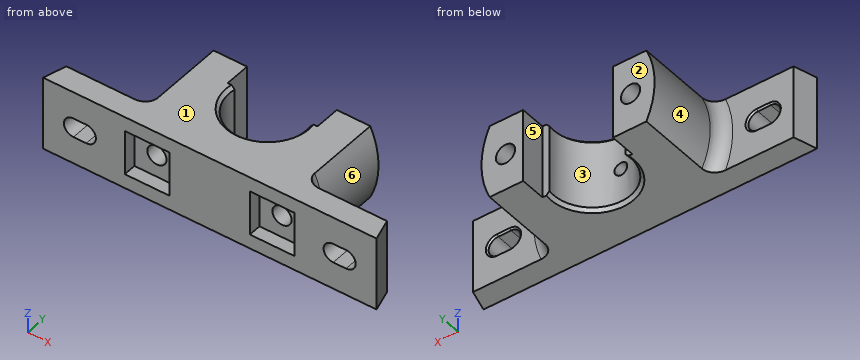
```python
from build123d import *

# Parameters (mm, degrees)
BOSS_EXTRUDE1_DEPTH = 23
BOSS_EXTRUDE2_DEPTH = 54
CUT_EXTRUDE1_DEPTH  = 47
SKETCH4_R           = 6
CUT_EXTRUDE2_DEPTH  = 69
SKETCH5_W           = 28
SKETCH5_H           = 28
CUT_EXTRUDE3_DEPTH  = 8
CUT_EXTRUDE4_DEPTH  = 15
SKETCH7_R           = 4
CUT_EXTRUDE5_DEPTH  = 54
FILLET1_R           = 8
CHAMFER1_SIZE       = 2
CHAMFER2_SIZE       = 1


with BuildPart() as part:
    # Sketch1 → Boss-Extrude1 (new body, symmetric)
    with BuildSketch(Plane.XY):
        Polygon((-104, 0), (104, 0), (99.985564599, 14), (-99.985564599, 14), align=None)
    extrude(amount=BOSS_EXTRUDE1_DEPTH, both=True)

    # Sketch2 → Boss-Extrude2 (add)
    with BuildSketch(Plane(origin=(0, 14, 0), x_dir=(1, 0, 0), z_dir=(0, 1, 0))):
        with BuildLine():
            Line((48.856934001, 23), (-48.856934001, 23))
            ThreePointArc((-48.856934001, 23), (-54, 0), (-48.856934001, -23))
            Line((-48.856934001, -23), (48.856934001, -23))
            ThreePointArc((48.856934001, -23), (54, 0), (48.856934001, 23))
        make_face()
    extrude(amount=BOSS_EXTRUDE2_DEPTH)

    # Sketch3 → Cut-Extrude1 (cut, through all)
    with BuildSketch(Plane.XY.offset(23)):
        with BuildLine():
            Line((-28, 68), (-28, 52))
            Line((-28, 52), (-23.664319132, 52))
            ThreePointArc((-23.664319132, 52), (0, 24), (23.664319132, 52))
            Line((23.664319132, 52), (28, 52))
            Line((28, 52), (28, 68))
            Line((28, 68), (-28, 68))
        make_face()
    extrude(amount=-CUT_EXTRUDE1_DEPTH, mode=Mode.SUBTRACT)

    # Sketch4 → Cut-Extrude2 (cut, through all)
    with BuildSketch(Plane(origin=(0, 68, 0), x_dir=(1, 0, 0), z_dir=(0, 1, 0))):
        with Locations(Location((-39, 0, 0), (0, 0, 270))):  # turned: the seam where the file's is
            Circle(SKETCH4_R)
        with Locations(Location((39, 0, 0), (0, 0, 270))):  # turned: the seam where the file's is
            Circle(SKETCH4_R)
    extrude(amount=-CUT_EXTRUDE2_DEPTH, mode=Mode.SUBTRACT)

    # Sketch5 → Cut-Extrude3 (cut)
    with BuildSketch(Plane.XZ):
        with Locations((-39, 0)):
            Rectangle(SKETCH5_W, SKETCH5_H)
        with Locations((39, 0)):
            Rectangle(SKETCH5_W, SKETCH5_H)
    extrude(amount=-CUT_EXTRUDE3_DEPTH, mode=Mode.SUBTRACT)

    # Sketch6 → Cut-Extrude4 (cut, through all)
    with BuildSketch(Plane(origin=(0, 14, 0), x_dir=(1, 0, 0), z_dir=(0, 1, 0))):
        with BuildLine():
            Line((-85, 6), (-77, 6))
            ThreePointArc((-77, 6), (-71, 0), (-77, -6))
            Line((-77, -6), (-85, -6))
            ThreePointArc((-85, -6), (-91, 0), (-85, 6))
        make_face()
    cut_extrude4 = extrude(amount=-CUT_EXTRUDE4_DEPTH, mode=Mode.SUBTRACT)

    # Mirror1: Cut-Extrude4 across plane
    add(cut_extrude4.mirror(Plane(origin=(0, 0, 0), x_dir=(0, 0, 1), z_dir=(1, 0, 0))), mode=Mode.SUBTRACT)

    # Sketch7 → Cut-Extrude5 (cut)
    with BuildSketch(Plane(origin=(0, 68, 0), x_dir=(1, 0, 0), z_dir=(0, 1, 0))):
        with Locations(Location((0, 0, 0), (0, 0, 270))):  # turned: the seam where the file's is
            Circle(SKETCH7_R)
    extrude(amount=-CUT_EXTRUDE5_DEPTH, mode=Mode.SUBTRACT)

    # Fillet1
    fillet1_edges = [part.edges().sort_by_distance(p)[0] for p in [
        (54, 14, 0),
        (-54, 14, 0),
    ]]
    fillet(fillet1_edges, radius=FILLET1_R)

    # Chamfer1
    chamfer1_edges = [part.edges().sort_by_distance(p)[0] for p in [
        (0, 24, -23),
        (0, 24, 23),
    ]]
    chamfer(chamfer1_edges, length=CHAMFER1_SIZE)

    # Chamfer2
    chamfer2_edges = [part.edges().sort_by_distance(p)[0] for p in [
        (91, 14, 0),
        (81, 14, 6),
        (71, 14, 0),
        (81, 14, -6),
        (-91, 14, 0),
        (-81, 14, 6),
        (-71, 14, 0),
        (-81, 14, -6),
    ]]
    chamfer(chamfer2_edges, length=CHAMFER2_SIZE)


solid = part.part
```
The listing builds one solid part. Answer for the finished solid, in the listing's coordinates (mm). Face numbers are marked on the shaded views. A direction names the side the tool comes from. Round coordinates to 2 decimals unless told otherwise and drop trailing zeros. Write each loop counter-clockwise with the first axis right and the second up, starting at its lowest first coordinate (ties: lowest second). Pieces come first, ordered by that corner, then holes. Notation, with made-up numbers: (-16.5, -22) -> (15.5, -22) arc R26 cw to (15.5, 2) -> close; hole circle Ø5 at (-34.75, -3.75). An arc over 180 degrees is marked (long way). Write item = value, one per line.
1) Which of the six approach directions +Z, -Z, +X, -X, +Y, -Y give full straight-line access (tool end or side, diameter ignored) to the marked faces 4, 5 and 6?
Check values:
face_4 = -X, +Y
face_5 = +Z, -Z, +Y
face_6 = +X, +Y
2) Given pin 1 (1.5 mm diameter, centred on x = 22, z = 6.5, fed in from -Y); pin 2 (4 mm diameter, centred on y = 5.5, z = 5, fed in from -X); pin 3 (14 mm diameter, centred on x = -39, z = 0, fed in from -Y); pin 4 (8 mm diameter, centred on x = 39, z = 0, fed in from -Y), each flat-ended and moving along its own axis, determine where each tip first touches the part or whether it passes through.
Check values:
pin_1 = 0
pin_2 = -103
pin_3 = 8
pin_4 = through
3) Section A-A on y = 48 is taken. Write down the section's boundary in (x, z), plus the area to 3 significant figures.
Check values:
outline = (-48.86, -23) -> (-26, -23) -> (-24, -21) -> (-24, 21) -> (-26, 23) -> (-48.86, 23) arc R54 ccw to start; (24, -21) -> (26, -23) -> (48.86, -23) arc R54 ccw to (48.86, 23) -> (26, 23) -> (24, 21) -> close; hole circle Ø12 at (-39, 0); hole circle Ø12 at (39, 0)
area = 2,370 mm²
4) Straight lines are drawn through the part: line 1 along X through (y, z) = (22.5, 0.5); line 2 along X through (y, z) = (28.5, 2); line 3 along Y through (x, z) = (-7, -6.5). For each, find the intervals that lie inside material, in ascending order. Write a range as [from, to].
Check values:
line_1 = [-54, -44.98], [-33.02, -3.97], [3.97, 33.02], [44.98, 54]
line_2 = [-53.96, -44.66], [-33.34, -13.99], [13.99, 33.34], [44.66, 53.96]
line_3 = [0, 25.04]
5) For a pull along Y with two mould halves and no side action, classify the marked faces 1, 2 and 3 as released by +Y, released by -Y, zero draft, split by the parting line, or undercut.
Check values:
face_1 = zero draft
face_2 = released by +Y
face_3 = undercut
6) Section B-B on x = -39 is taken. Write down the section's boundary in (y, z).
Check values:
outline = (0, -23) -> (68, -23) -> (68, -6) -> (8, -6) -> (8, -14) -> (0, -14) -> close; (0, 14) -> (8, 14) -> (8, 6) -> (68, 6) -> (68, 23) -> (0, 23) -> close
7) Section C-C on x = 0 is taken. Write down the section's boundary in (y, z), plus the area to 3 significant figures.
Check values:
outline = (0, -23) -> (22, -23) -> (24, -21) -> (24, -4) -> (14, -4) -> (14, 4) -> (24, 4) -> (24, 21) -> (22, 23) -> (0, 23) -> close
area = 1,020 mm²
8) Section D-D on z = 0 is taken. Give the number of separate pieces and of enclosed holes in the cut face, plus the area to 3 significant figures.
Check values:
separate_pieces = 5
enclosed_holes = 0
area = 4,190 mm²
